The listing builds one solid part. Answer for the finished solid, in the listing's coordinates (mm). Face numbers are marked on the shaded views. A direction names the side the tool comes from. Round coordinates to 2 decimals unless told otherwise and drop trailing zeros. Write each loop counter-clockwise with the first axis right and the second up, starting at its lowest first coordinate (ties: lowest second). Pieces come first, ordered by that corner, then holes. Notation, with made-up numbers: M 83.25,11 L 130.25,11 A17 cw 130.25,19 Z; hole C 25,18 d10. An arc over 180 degrees is marked long. Write each question's results on one line, items separated by ' | '.
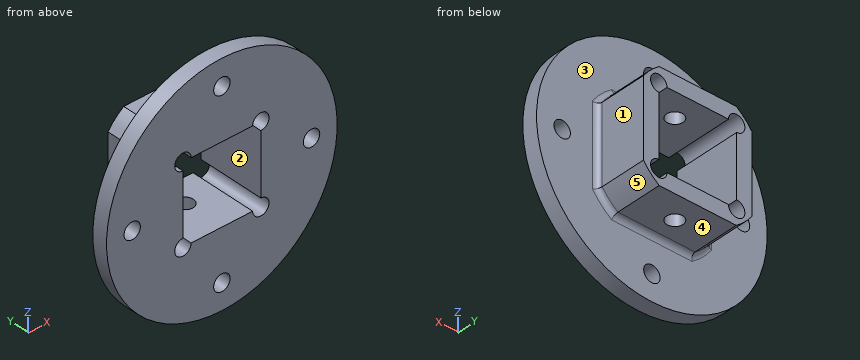
from build123d import *

# Parameters (mm, degrees)
SKETCH_1_R          = 22.5
SKETCH_1_R_2        = 1.6
SKETCH_1_W          = 15.2
SKETCH_1_H          = 15.2
EXTRUDE_1_DEPTH     = 3
SKETCH_2_W          = 15.2
SKETCH_2_H          = 15.2
EXTRUDE_2_DEPTH     = 10
SKETCH_3_R          = 1.6
CUT_EXTRUDE_1_DEPTH = 43.081587423
FILLET_1_R          = 1
SKETCH_4_R          = 1.6
CUT_EXTRUDE_2_DEPTH = 35.372954485


with BuildPart() as part:
    # 草图1 → 凸台-拉伸1 (new body)
    with BuildSketch(Plane(origin=(0, 0, 0), x_dir=(1, 0, 0), z_dir=(0, 1, 0))):
        with Locations(Location((0, 0, 0), (0, 0, 270))):
            Circle(SKETCH_1_R)
        with Locations(Location((0, 17.5, 0), (0, 0, 270))):
            Circle(SKETCH_1_R_2, mode=Mode.SUBTRACT)
        with Locations(Location((17.5, 0, 0), (0, 0, 270))):
            Circle(SKETCH_1_R_2, mode=Mode.SUBTRACT)
        with Locations(Location((0, -17.5, 0), (0, 0, 270))):
            Circle(SKETCH_1_R_2, mode=Mode.SUBTRACT)
        with Locations(Location((-17.5, 0, 0), (0, 0, 270))):
            Circle(SKETCH_1_R_2, mode=Mode.SUBTRACT)
        Rectangle(SKETCH_1_W, SKETCH_1_H, mode=Mode.SUBTRACT)
    extrude(amount=EXTRUDE_1_DEPTH)

    # 草图2 → 凸台-拉伸2 (add)
    with BuildSketch(Plane(origin=(0, 3, 0), x_dir=(1, 0, 0), z_dir=(0, 1, 0))):
        with BuildLine():
            Line((-10.6, -7.525955089), (-10.6, 7.525955089))
            ThreePointArc((-10.6, 7.525955089), (-9.192388155, 9.192388155), (-7.525955089, 10.6))
            Line((-7.525955089, 10.6), (7.525955089, 10.6))
            ThreePointArc((7.525955089, 10.6), (9.192388155, 9.192388155), (10.6, 7.525955089))
            Line((10.6, 7.525955089), (10.6, -7.525955089))
            ThreePointArc((10.6, -7.525955089), (9.192388155, -9.192388155), (7.525955089, -10.6))
            Line((7.525955089, -10.6), (-7.525955089, -10.6))
            ThreePointArc((-7.525955089, -10.6), (-9.192388155, -9.192388155), (-10.6, -7.525955089))
        make_face()
        Rectangle(SKETCH_2_W, SKETCH_2_H, mode=Mode.SUBTRACT)
    extrude(amount=EXTRUDE_2_DEPTH)

    # 草图3 → 切除-拉伸1 (cut, through all)
    with BuildSketch(Plane(origin=(0, 0, -10.6), x_dir=(-1, 0, 0), z_dir=(0, 0, -1))):
        with Locations((0, 8)):
            Circle(SKETCH_3_R)
    extrude(amount=-CUT_EXTRUDE_1_DEPTH, mode=Mode.SUBTRACT)

    # 圆角1
    fillet_1_edges = [part.edges().sort_by_distance(p)[0] for p in [
        (9.192388155, 3, 9.192388155),
        (10.6, 3, 0),
        (9.192388155, 3, -9.192388155),
        (0, 3, -10.6),
        (-9.192388155, 3, -9.192388155),
        (-10.6, 3, 0),
        (-9.192388155, 3, 9.192388155),
        (0, 3, 10.6),
    ]]
    fillet(fillet_1_edges, radius=FILLET_1_R)

    # 草图4 → 切除-拉伸2 (cut, through all)
    with BuildSketch(Plane(origin=(0, 13, 0), x_dir=(1, 0, 0), z_dir=(0, 1, 0))):
        with Locations((7.6, 7.6)):
            Circle(SKETCH_4_R)
        with Locations((7.6, -7.6)):
            Circle(SKETCH_4_R)
        with Locations((-7.6, -7.6)):
            Circle(SKETCH_4_R)
        with Locations((-7.6, 7.6)):
            Circle(SKETCH_4_R)
    extrude(amount=-CUT_EXTRUDE_2_DEPTH, mode=Mode.SUBTRACT)


solid = part.part
1) Section B-B (z = 0) is taken. Determine the outline of the cut face in (x, y).
Return value:
outline: M -22.5,0 L -19.1,0 L -19.1,3 L -22.5,3 Z; M -15.9,0 L -7.6,0 L -7.6,13 L -10.6,13 L -10.6,4 A1 cw -11.6,3 L -15.9,3 Z; M 7.6,0 L 15.9,0 L 15.9,3 L 11.6,3 A1 cw 10.6,4 L 10.6,13 L 7.6,13 Z; M 19.1,0 L 22.5,0 L 22.5,3 L 19.1,3 Z
2) Each of these flat-tipped pins is pushed along its axis until it touches: pin 1 (6 mm diameter, centred on y = 7.5, z = -1, fed in from -X); pin 2 (1 mm diameter, centred on x = -1, z = -15.5, fed in from +Y); pin 3 (6 mm diameter, centred on y = 10.5, z = -4, fed in from +X). Where does it stop, or does it pass through?
Return value:
pin 1: x = -10.6 | pin 2: y = 3 | pin 3: x = 10.6
3) A tool of negligible diameter and unlimited length cuts with its end or side. For the marked faces 1, 2, 3, 4 and 5, from which of +Z, -Z, +X, -X, +Y, -Y can it reach the whole face along a straight path? Write none if from no direction.
Return value:
face 1: +Z, -Z, +X, +Y | face 2: +Y, -Y | face 3: +Y | face 4: -Z, +X, -X, +Y | face 5: -Z, +X, +Y
4) Section C-C (x = 0) is taken. State how many separate pieces and enclosed holes the cut face has, then the cut area to 3 significant figures.
Return value:
separate pieces: 6 | enclosed holes: 0 | area: 111 mm²
5) Section A-A (y = 10.5) is taken. Determine the outline of the cut face in (x, z), then the cut area to 3 significant figures.
Return value:
outline: M -10.6,-7.53 A13 ccw -7.53,-10.6 L 7.53,-10.6 A13 ccw 10.6,-7.53 L 10.6,7.53 A13 ccw 7.53,10.6 L -7.53,10.6 A13 ccw -10.6,7.53 Z; hole M -7.6,-6 A1.6 ccw long -6,-7.6 L 6,-7.6 A1.6 ccw long 7.6,-6 L 7.6,6 A1.6 ccw long 6,7.6 L -6,7.6 A1.6 ccw long -7.6,6 Z | area: 177 mm²
6) Section D-D (y = 8) is taken. Determine the outline of the cut face in (x, z).
Return value:
outline: M -10.6,-7.53 A13 ccw -7.53,-10.6 L -1.6,-10.6 L -1.6,-7.6 L -6,-7.6 A1.6 cw long -7.6,-6 L -7.6,6 A1.6 cw long -6,7.6 L -1.6,7.6 L -1.6,10.6 L -7.53,10.6 A13 ccw -10.6,7.53 Z; M 1.6,-10.6 L 7.53,-10.6 A13 ccw 10.6,-7.53 L 10.6,7.53 A13 ccw 7.53,10.6 L 1.6,10.6 L 1.6,7.6 L 6,7.6 A1.6 cw long 7.6,6 L 7.6,-6 A1.6 cw long 6,-7.6 L 1.6,-7.6 Z
7) Find the intervals of material crossed by line 1 (X direction, y = 1.15, z = 0); line 2 (Z direction, x = 9, y = 9.75); line 3 (Y direction, x = 4.5, z = 13), in increasing order.
Return value:
line 1: -22.5 to -19.1, -15.9 to -7.6, 7.6 to 15.9, 19.1 to 22.5 | line 2: -9.38 to -8.37, -6.83 to 6.83, 8.37 to 9.38 | line 3: 0 to 3
